Source: CAD feature listing. Evaluate the final solid. Frame: model axes, mm. Face numbers are marked on the shaded views. A direction names the side the tool comes from. Round coordinates to 2 decimals unless told otherwise and drop trailing zeros. Order: outer loops, then holes, each group sorted by start corner. A loop starts at its lowest first (then second) coordinate and runs counter-clockwise, first axis right, second up. Notation, with made-up numbers: (-24.5, 31.5) -> (-11.5, 31.5) arc R19 cw to (-11.5, 55.5) -> close; hole circle Ø3 at (83, -17). An arc over 180 degrees is marked (long way). Write item = value, one per line. Start each with the question number.
(1) Reachability of the marked faces 4, 5 and 6 from +Z, -Z, +X, -X, +Y, -Y: full face, straight path, thin tool, end or side. Return the list, or none.
(2) Contact query for flat-ended pins moving along their axis: pin 1 Ø13 at (x, z) = (92, -20.5) entering from +Y; pin 2 Ø8 at (y, z) = (91, 10) entering from +X; pin 3 Ø4 at (y, z) = (76, 10) entering from -X; pin 4 Ø2 at (x, y) = (89.5, 16.5) entering from -Z. Output: stop coordinate, or through.
(3) Ray query, line 1 (Y direction, x = 131, z = 128); line 2 (Y direction, x = -113.2, z = 10); line 3 (X direction, y = 26.5, z = 60.5). Return the intervals inside material, ascending.
(4) Draft query along X for the marked faces 1, 2 and 3. Return one class per face: released by +X, released by -X, zero draft, split by the parting line, or undercut.
(5) Cut plane A-A on x = -9. Return the cut outline in (y, z), then the cut area to 3 significant figures.
from build123d import *

# Parameters (mm, degrees)
SM_START                           = -110
SM_BASE_FLANGE_1_DEPTH             = 220
SKETCH_6_R                         = 17.5
CUT_EXTRUDE_1_DEPTH                = 10
HOLE_WIZARD_7_0_7_1_D              = 7
SKETCH_21_W                        = 100
SKETCH_21_H                        = 11
CUT_EXTRUDE_4_DEPTH                = 153.318744743
FILLET_1_R                         = 10
SM_EDGE_FLANGE_1_DEPTH             = 85
SM_EDGE_FLANGE_1_BEND_DEPTH        = 85
SM_EDGE_FLANGE_2_STRIP_W           = 12.8
SM_EDGE_FLANGE_2_STRIP_H           = 2
SM_EDGE_FLANGE_2_STRIP_CUT_DEPTH   = 85
SM_EDGE_FLANGE_2_STRIP_2_W         = 12.8
SM_EDGE_FLANGE_2_STRIP_2_H         = 2
SM_EDGE_FLANGE_2_STRIP_CUT_2_DEPTH = 85
SM_EDGE_FLANGE_2_DEPTH             = 85
SM_EDGE_FLANGE_2_BEND_DEPTH        = 85
FILLET_2_R                         = 10
CUT_EXTRUDE_5_DEPTH                = 304.981726424
CUT_EXTRUDE_6_DEPTH                = 10
HOLE_WIZARD_7_0_7_2_D              = 7
HOLE_WIZARD_7_0_7_2_DEPTH          = 14
HOLE_WIZARD_7_0_7_2_TIP            = 2.103012167
F_7_0_7_DIAMETER_HOLE1_AT_2_COUNT  = 2
F_7_0_7_DIAMETER_HOLE1_AT_2_PITCH  = 15
F_10_5_10_5_DIAMETER_HOLE1_D       = 10.5


# Read off the part's stored shape, not the designer's step: Базовая кромка1
# Sheet-metal steps are written as plain solids
with BuildPart() as part:
    # Базовая кромка1 outline → Базовая кромка1 (new body)
    with BuildSketch(Plane(origin=(0, 0, 0), x_dir=(0, 0, -1), z_dir=(1, 0, 0)).offset(SM_START)):
        with BuildLine():
            Line((4.4, 0), (30, 0))
            Line((30, 0), (30, 2))
            Line((30, 2), (4.4, 2))
            ThreePointArc((4.4, 2), (2.702943725, 2.702943725), (2, 4.4))
            Line((2, 4.4), (2, 101))
            Line((2, 101), (0, 101))
            Line((0, 101), (0, 4.4))
            ThreePointArc((0, 4.4), (1.288730163, 1.288730163), (4.4, 0))
        make_face()
    extrude(amount=SM_BASE_FLANGE_1_DEPTH)

    # Эскиз6 → Вырез-Вытянуть1 (cut)
    with BuildSketch(Plane.XY):
        with Locations((0, 44)):
            Circle(SKETCH_6_R)
    extrude(amount=-CUT_EXTRUDE_1_DEPTH, mode=Mode.SUBTRACT)

    # Диаметр отверстия Ø7.0 (7)1 (through all)
    with Locations(Plane(origin=(0, 0, 0), x_dir=(-1, 0, 0), z_dir=(0, -1, 0))):
        with Locations((95, 20), (65, 20), (-65, 20), (-95, 20)):
            Hole(HOLE_WIZARD_7_0_7_1_D / 2)

    # Эскиз21 → Вырез-Вытянуть4 (cut, through all)
    with BuildSketch(Plane.XY):
        with Locations((0, 5.5)):
            Rectangle(SKETCH_21_W, SKETCH_21_H)
    extrude(amount=-CUT_EXTRUDE_4_DEPTH, mode=Mode.SUBTRACT)

    # Скругление1
    fillet_1_edges = [part.edges().sort_by_distance(p)[0] for p in [
        (110, 1, -30),
        (-50, 1, -30),
        (50, 1, -30),
        (-110, 1, -30),
    ]]
    fillet(fillet_1_edges, radius=FILLET_1_R)

    # Ребро-кромка1 section (across the edge) → Ребро-кромка1 (add)
    with BuildSketch(Plane(origin=(112.4, 16, 0), x_dir=(-1, 0, 0), z_dir=(0, 1, 0))):
        with BuildLine():
            Line((-2, 2.4), (-2, 129.5))
            Line((-2, 129.5), (0, 129.5))
            Line((0, 129.5), (0, 2.4))
            ThreePointArc((0, 2.4), (0.702943725, 0.702943725), (2.4, 0))
            Line((2.4, 0), (2.4, -2))
            ThreePointArc((2.4, -2), (-0.711269837, -0.711269837), (-2, 2.4))
        make_face()
    extrude(amount=SM_EDGE_FLANGE_1_DEPTH)

    # Ребро-кромка1 section 2 (across the edge) → Ребро-кромка1 bend (add)
    with BuildSketch(Plane(origin=(-112.4, 101, 0), x_dir=(1, 0, 0), z_dir=(0, -1, 0))):
        with BuildLine():
            Line((-2, 2.4), (-2, 129.5))
            Line((-2, 129.5), (0, 129.5))
            Line((0, 129.5), (0, 2.4))
            ThreePointArc((0, 2.4), (0.702943725, 0.702943725), (2.4, 0))
            Line((2.4, 0), (2.4, -2))
            ThreePointArc((2.4, -2), (-0.711269837, -0.711269837), (-2, 2.4))
        make_face()
    extrude(amount=SM_EDGE_FLANGE_1_BEND_DEPTH)

    # Ребро-кромка2 strip (across the edge) → Ребро-кромка2 strip cut (cut)
    with BuildSketch(Plane(origin=(114.4, 101, 129.5), x_dir=(0, 0, -1), z_dir=(0, -1, 0))):
        with Locations((-2, -1)):
            Rectangle(SM_EDGE_FLANGE_2_STRIP_W, SM_EDGE_FLANGE_2_STRIP_H)
    extrude(amount=SM_EDGE_FLANGE_2_STRIP_CUT_DEPTH, mode=Mode.SUBTRACT)

    # Ребро-кромка2 strip 2 (across the edge) → Ребро-кромка2 strip cut 2 (cut)
    with BuildSketch(Plane(origin=(-114.4, 16, 129.5), x_dir=(0, 0, -1), z_dir=(0, 1, 0))):
        with Locations((-2, -1)):
            Rectangle(SM_EDGE_FLANGE_2_STRIP_2_W, SM_EDGE_FLANGE_2_STRIP_2_H)
    extrude(amount=SM_EDGE_FLANGE_2_STRIP_CUT_2_DEPTH, mode=Mode.SUBTRACT)

    # Ребро-кромка2 section (across the edge) → Ребро-кромка2 (add)
    with BuildSketch(Plane(origin=(114.4, 101, 129.5), x_dir=(0, 0, -1), z_dir=(0, -1, 0))):
        with BuildLine():
            Line((0, 2.4), (0, 27))
            Line((0, 27), (2, 27))
            Line((2, 27), (2, 2.4))
            ThreePointArc((2, 2.4), (2.702943725, 0.702943725), (4.4, 0))
            Line((4.4, 0), (4.4, -2))
            ThreePointArc((4.4, -2), (1.288730163, -0.711269837), (0, 2.4))
        make_face()
    extrude(amount=SM_EDGE_FLANGE_2_DEPTH)

    # Ребро-кромка2 section 2 (across the edge) → Ребро-кромка2 bend (add)
    with BuildSketch(Plane(origin=(-114.4, 16, 129.5), x_dir=(0, 0, -1), z_dir=(0, 1, 0))):
        with BuildLine():
            Line((0, 2.4), (0, 27))
            Line((0, 27), (2, 27))
            Line((2, 27), (2, 2.4))
            ThreePointArc((2, 2.4), (2.702943725, 0.702943725), (4.4, 0))
            Line((4.4, 0), (4.4, -2))
            ThreePointArc((4.4, -2), (1.288730163, -0.711269837), (0, 2.4))
        make_face()
    extrude(amount=SM_EDGE_FLANGE_2_BEND_DEPTH)

    # Скругление2
    fillet_2_edges = [part.edges().sort_by_distance(p)[0] for p in [
        (141.4, 101, 128.5),
        (141.4, 16, 128.5),
        (-141.4, 16, 128.5),
        (-141.4, 101, 128.5),
    ]]
    fillet(fillet_2_edges, radius=FILLET_2_R)

    # Эскиз34 → Вырез-Вытянуть5 (cut, through all)
    with BuildSketch(Plane(origin=(114.4, 0, 0), x_dir=(0, 0, -1), z_dir=(1, 0, 0))):
        with BuildLine():
            Line((-107.1, 86), (-32.357951658, 86))
            ThreePointArc((-32.357951658, 86), (-29.416528086, 83.589938443), (-31.201112429, 80.232018245))
            Line((-31.201112429, 80.232018245), (-105.943160771, 48.99462536))
            ThreePointArc((-105.943160771, 48.99462536), (-108.762751081, 49.265557087), (-110.1, 51.762607115))
            Line((-110.1, 51.762607115), (-110.1, 83))
            ThreePointArc((-110.1, 83), (-109.221320344, 85.121320344), (-107.1, 86))
        make_face()
        with BuildLine():
            Line((-96.298887571, 36.767981755), (-21.556839229, 68.00537464))
            ThreePointArc((-21.556839229, 68.00537464), (-18.737248919, 67.734442913), (-17.4, 65.237392885))
            Line((-17.4, 65.237392885), (-17.4, 34))
            ThreePointArc((-17.4, 34), (-18.278679656, 31.878679656), (-20.4, 31))
            Line((-20.4, 31), (-95.142048342, 31))
            ThreePointArc((-95.142048342, 31), (-98.083471914, 33.410061557), (-96.298887571, 36.767981755))
        make_face()
    extrude(amount=-CUT_EXTRUDE_5_DEPTH, mode=Mode.SUBTRACT)

    # Эскиз35 → Вырез-Вытянуть6 (cut)
    with BuildSketch(Plane.XY):
        with BuildLine():
            Line((-70.404878533, 86), (-92, 86))
            ThreePointArc((-92, 86), (-94.121320344, 85.121320344), (-95, 83))
            Line((-95, 83), (-95, 45.596152423))
            ThreePointArc((-95, 45.596152423), (-92.776457135, 42.698374944), (-89.401923789, 44.096152423))
            Line((-89.401923789, 44.096152423), (-67.806802321, 81.5))
            ThreePointArc((-67.806802321, 81.5), (-67.806802321, 84.5), (-70.404878533, 86))
        make_face()
        with BuildLine():
            Line((95, 83), (95, 45.596152423))
            ThreePointArc((95, 45.596152423), (92.776457135, 42.698374944), (89.401923789, 44.096152423))
            Line((89.401923789, 44.096152423), (67.806802321, 81.5))
            ThreePointArc((67.806802321, 81.5), (67.806802321, 84.5), (70.404878533, 86))
            Line((70.404878533, 86), (92, 86))
            ThreePointArc((92, 86), (94.121320344, 85.121320344), (95, 83))
        make_face()
    extrude(amount=-CUT_EXTRUDE_6_DEPTH, mode=Mode.SUBTRACT)

    # Диаметр отверстия Ø7.0 (7)2
    with Locations(Plane.XY.offset(129.5)):
        with Locations((-131.4, 91), (-131.4, 26), (131.4, 91), (131.4, 26)):
            Hole(HOLE_WIZARD_7_0_7_2_D / 2, depth=HOLE_WIZARD_7_0_7_2_DEPTH)
            with Locations((0, 0, -(HOLE_WIZARD_7_0_7_2_DEPTH + HOLE_WIZARD_7_0_7_2_TIP / 2))):  # 118° drill point
                Cone(0, HOLE_WIZARD_7_0_7_2_D / 2, HOLE_WIZARD_7_0_7_2_TIP, mode=Mode.SUBTRACT)

    # Эскиз40 → Ø7.0 (7) Diameter Hole1 (revolve, cut)
    with BuildSketch(Plane(origin=(114.4, 91, 10), x_dir=(0, 0, -1), z_dir=(0, 1, 0))):
        Polygon((0, 0), (0, 7.103012167), (3.5, 5), (3.5, 0), align=None)
    f_7_0_7_diameter_hole1 = revolve(axis=Axis((120.75, 91, 10), (-1, 0, 0)), mode=Mode.SUBTRACT)

    # Ø7.0 (7) Diameter Hole1 at 2: Ø7.0 (7) Diameter Hole1 ×2
    with Locations(*[(0, -i * F_7_0_7_DIAMETER_HOLE1_AT_2_PITCH, 0) for i in range(1, F_7_0_7_DIAMETER_HOLE1_AT_2_COUNT)]):
        add(f_7_0_7_diameter_hole1, mode=Mode.SUBTRACT)

    # Зеркальное отражение1: Ø7.0 (7) Diameter Hole1 across plane
    add(f_7_0_7_diameter_hole1.mirror(Plane(origin=(0, 0, 0), x_dir=(0, 0, 1), z_dir=(1, 0, 0))), mode=Mode.SUBTRACT)

    # Зеркальное отражение1 copy 1 sketch → Зеркальное отражение1 copy 1 (revolve, cut)
    with BuildSketch(Plane(origin=(-114.4, 76, 10), x_dir=(0, 0, -1), z_dir=(0, 1, 0))):
        Polygon((0, 0), (0, -7.103012167), (3.5, -5), (3.5, 0), align=None)
    revolve(axis=Axis((-120.75, 76, 10), (-1, 0, 0)), mode=Mode.SUBTRACT)

    # Ø10.5 (10.5) Diameter Hole1 (through all)
    with Locations(Plane(origin=(0, 0, -2), x_dir=(-1, 0, 0), z_dir=(0, 0, -1))):
        with Locations((-58.5, 44), (58.5, 44)):
            Hole(F_10_5_10_5_DIAMETER_HOLE1_D / 2)


solid = part.part
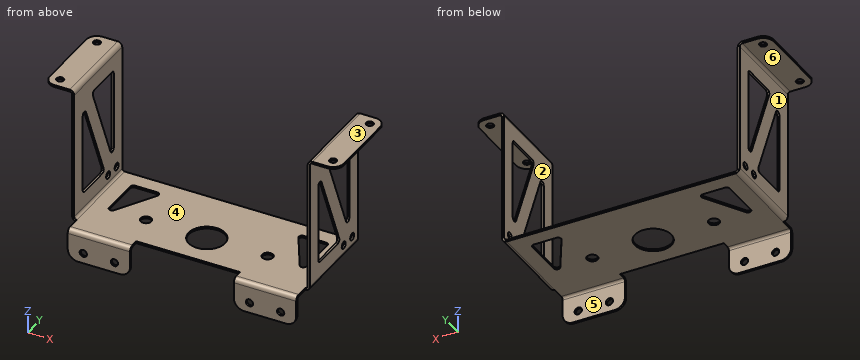
Evaluation:
q1.face_4 = +Z, +Y, -Y
q1.face_5 = -Z, +X, -X, +Y
q1.face_6 = -Z, -X, +Y, -Y
q2.pin_1 = 2
q2.pin_2 = 114.4
q2.pin_3 = through
q2.pin_4 = -2
q3.line_1 = 16 to 22.52, 29.48 to 87.52, 94.48 to 101
q3.line_2 = 16 to 72.5, 79.5 to 87.5, 94.5 to 101
q3.line_3 = -114.4 to -112.4, 112.4 to 114.4
q4.face_1 = released by -X
q4.face_2 = undercut
q4.face_3 = zero draft
q5.outline = (11, -2) -> (28.99, -2) -> (28.99, 0) -> (11, 0) -> close; (59.01, -2) -> (101, -2) -> (101, 0) -> (59.01, 0) -> close
q5.area = 120 mm^2
